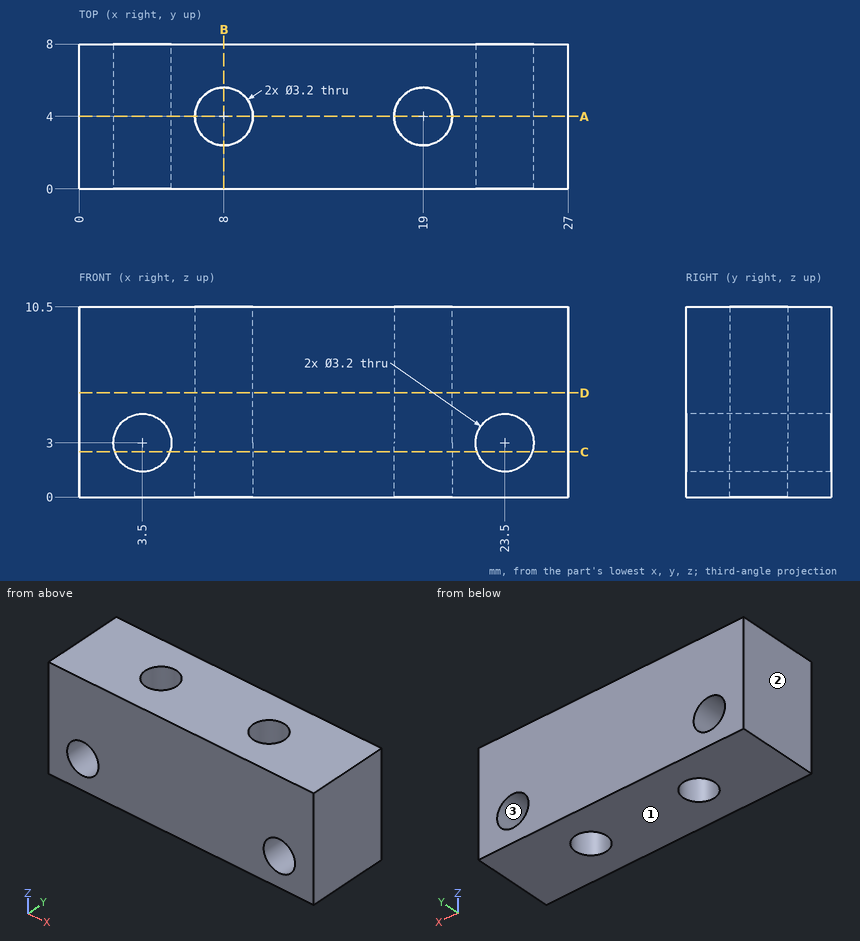
The drawing under review shows one solid part. Ordinate dimensions are in mm from its lowest x, y, z. Give positions to 0.01 mm unless a question says otherwise; leave off trailing zeros. Order: outer loops, then holes, each group sorted by start corner. A loop starts at its lowest first (then second) coordinate and runs counter-clockwise, first axis right, second up. Notation, with made-up numbers: (-32, 83.25) -> (1, 83.25) arc R17 cw to (1, 98.25) -> close; hole circle Ø2 at (25, 26.25). An arc over 180 degrees is marked (long way). Write item = value, one per line.
1) We need section C-C, the plane z = 2.5. Give the boundary of the cut face in (x, y), and give its area (3 significant figures).
Findings:
outline = (0, 0) -> (1.98, 0) -> (1.98, 8) -> (0, 8) -> close; (5.02, 0) -> (21.98, 0) -> (21.98, 8) -> (5.02, 8) -> close; (25.02, 0) -> (27, 0) -> (27, 8) -> (25.02, 8) -> close; hole circle Ø3.2 at (8, 4); hole circle Ø3.2 at (19, 4)
area = 151 mm^2
2) To check wall thickness, follow L1, parallel to X at y = 4, z = 7.5; L2, parallel to Z at x = 3.5, y = 3.25; L3, parallel to X at y = 6.75, z = 3.5. State the ranges of each line that lie inside material, in increasing order. Write a range as from..to.
Findings:
L1 = 0..6.4, 9.6..17.4, 20.6..27
L2 = 0..1.4, 4.6..10.5
L3 = 0..1.98, 5.02..21.98, 25.02..27
3) We need section B-B, the plane x = 8. Give the boundary of the cut face in (y, z), and give its area (3 significant figures).
Findings:
outline = (0, 0) -> (2.4, 0) -> (2.4, 10.5) -> (0, 10.5) -> close; (5.6, 0) -> (8, 0) -> (8, 10.5) -> (5.6, 10.5) -> close
area = 50.4 mm^2
4) Draft analysis for pull direction Z (two halves, no side actions). For the marked faces 1, 2 and 3, state which applies: pulls with the +Z half, pulls with the -Z half, needs draft (parallel to the pull), parting line crosses it, or undercut.
Findings:
face_1 = pulls with the -Z half
face_2 = needs draft
face_3 = undercut
5) Insertion check: pin 1 (1.9 mm diameter, centred on x = 8, y = 4, fed in from +Z). The pin has a flat end and moves straight along its axis. Give the tip position at first contact, or say it passes through.
Findings:
pin_1 = through
6) We need section D-D, the plane z = 5.75. Give the boundary of the cut face in (x, y), and give its area (3 significant figures).
Findings:
outline = (0, 0) -> (27, 0) -> (27, 8) -> (0, 8) -> close; hole circle Ø3.2 at (8, 4); hole circle Ø3.2 at (19, 4)
area = 200 mm^2
7) We need section A-A, the plane y = 4. Give the boundary of the cut face in (x, z).
Findings:
outline = (0, 0) -> (6.4, 0) -> (6.4, 10.5) -> (0, 10.5) -> close; (9.6, 0) -> (17.4, 0) -> (17.4, 10.5) -> (9.6, 10.5) -> close; (20.6, 0) -> (27, 0) -> (27, 10.5) -> (20.6, 10.5) -> close; hole circle Ø3.2 at (3.5, 3); hole circle Ø3.2 at (23.5, 3)
